Source: CAD feature listing. Evaluate the final solid. Frame: model axes, mm. Give positions to 0.01 mm unless a question says otherwise; leave off trailing zeros. Write each loop counter-clockwise with the first axis right and the second up, starting at its lowest first coordinate (ties: lowest second). Pieces come first, ordered by that corner, then holes. Notation, with made-up numbers: (42, 8.5) -> (82, 8.5) arc R8 ccw to (82, 17.5) -> close; hole circle Ø9 at (-4, 76.5). An arc over 180 degrees is marked (long way). Answer as a JSON object with one key per item and string values. Group by question number.
Item 1: Section query B-B on y = 1.15. Return the cut outline in (x, z), plus the area to 3 significant figures.
Item 2: Pull-direction query (Z, two-part tool) for faces 1 (the face through (-43, 2.54, -5)), 2 (the face through (-52.846, 1.288, 24.946)), 3 (the face through (-0.84, 1.25, -38.09)), 4 (the face through (-52.846, 1.288, 63.046)); classes: pulls with the +Z half, pulls with the -Z half, needs draft (parallel to the pull), parting line crosses it, or undercut.
Item 3: Section query D-D on x = 0. Return the cut outline in (y, z), plus the area to 3 significant figures.
Item 4: First-contact query: pin 1 Ø6.5 at (x, z) = (-50.8, 50.8) entering from +Y; pin 2 Ø0.8 at (x, y) = (54.5, 1) entering from +Z. Flat tips, straight axial feed; report the tip coordinate or a pass-through.
Item 5: Section query C-C on z = 45. Return the cut outline in (x, y).
Item 6: Section query A-A on z = 5. Return the cut outline in (x, y).
Item 7: Ray query, probe 1 along X at (y, z) = (0.35, 63.5); probe 2 along X at (y, z) = (1.25, 2.5); probe 3 along X at (y, z) = (1.3, 26.5). Return the intervals inside material, ascending. Write a range as from..to.
from build123d import *

# Parameters (mm, degrees)
BOSS_EXTRUDE1_DEPTH = 2.54
SKETCH2_R           = 2.0955
CUT_EXTRUDE1_DEPTH  = 110.279053803


with BuildPart() as part:
    # Sketch1 → Boss-Extrude1 (new body)
    with BuildSketch(Plane(origin=(0, 0, 0), x_dir=(1, 0, 0), z_dir=(0, 1, 0))):
        with BuildLine():
            Line((-38.1, -88.9), (-38.1, 0))
            ThreePointArc((-38.1, 0), (0, 38.1), (38.1, 0))
            Line((38.1, 0), (38.1, -38.1))
            Line((38.1, -38.1), (63.5, -38.1))
            Line((63.5, -38.1), (63.5, 0))
            ThreePointArc((63.5, 0), (0, 63.5), (-63.5, 0))
            Line((-63.5, 0), (-63.5, -88.9))
            Line((-63.5, -88.9), (-38.1, -88.9))
        make_face()
    extrude(amount=BOSS_EXTRUDE1_DEPTH)

    # Sketch2 → Cut-Extrude1 (cut, through all)
    with BuildSketch(Plane(origin=(0, 2.54, 0), x_dir=(1, 0, 0), z_dir=(0, 1, 0))):
        with Locations(Location((-50.8, -76.2, 0), (0, 0, 270))):
            Circle(SKETCH2_R)
        with Locations(Location((-50.8, -63.5, 0), (0, 0, 270))):
            Circle(SKETCH2_R)
        with Locations(Location((-50.8, -50.8, 0), (0, 0, 270))):
            Circle(SKETCH2_R)
        with Locations(Location((-50.8, -38.1, 0), (0, 0, 270))):
            Circle(SKETCH2_R)
        with Locations(Location((-50.8, -25.4, 0), (0, 0, 270))):
            Circle(SKETCH2_R)
    extrude(amount=-CUT_EXTRUDE1_DEPTH, mode=Mode.SUBTRACT)


solid = part.part
Worked answers:
{
 "1": {"outline": "(-63.5, 0) arc R63.5 ccw to (63.5, 0) -> (63.5, 38.1) -> (38.1, 38.1) -> (38.1, 0) arc R38.1 cw to (-38.1, 0) -> (-38.1, 88.9) -> (-63.5, 88.9) -> close; hole circle Ø4.19 at (-50.8, 25.4); hole circle Ø4.19 at (-50.8, 38.1); hole circle Ø4.19 at (-50.8, 50.8); hole circle Ø4.19 at (-50.8, 63.5); hole circle Ø4.19 at (-50.8, 76.2)", "area": "7,210 mm^2"},
 "2": {"face 1": "needs draft", "face 2": "undercut", "face 3": "pulls with the +Z half", "face 4": "undercut"},
 "3": {"outline": "(0, -63.5) -> (2.54, -63.5) -> (2.54, -38.1) -> (0, -38.1) -> close", "area": "64.5 mm^2"},
 "4": {"pin 1": "y = 2.54", "pin 2": "z = 38.1"},
 "5": {"outline": "(-63.5, 0) -> (-38.1, 0) -> (-38.1, 2.54) -> (-63.5, 2.54) -> close"},
 "6": {"outline": "(-63.5, 0) -> (-38.1, 0) -> (-38.1, 2.54) -> (-63.5, 2.54) -> close; (38.1, 0) -> (63.5, 0) -> (63.5, 2.54) -> (38.1, 2.54) -> close"},
 "7": {"probe 1": "-63.5..-52.9, -48.7..-38.1", "probe 2": "-63.5..-38.1, 38.1..63.5", "probe 3": "-63.5..-52.58, -49.02..-38.1, 38.1..63.5"}
}
